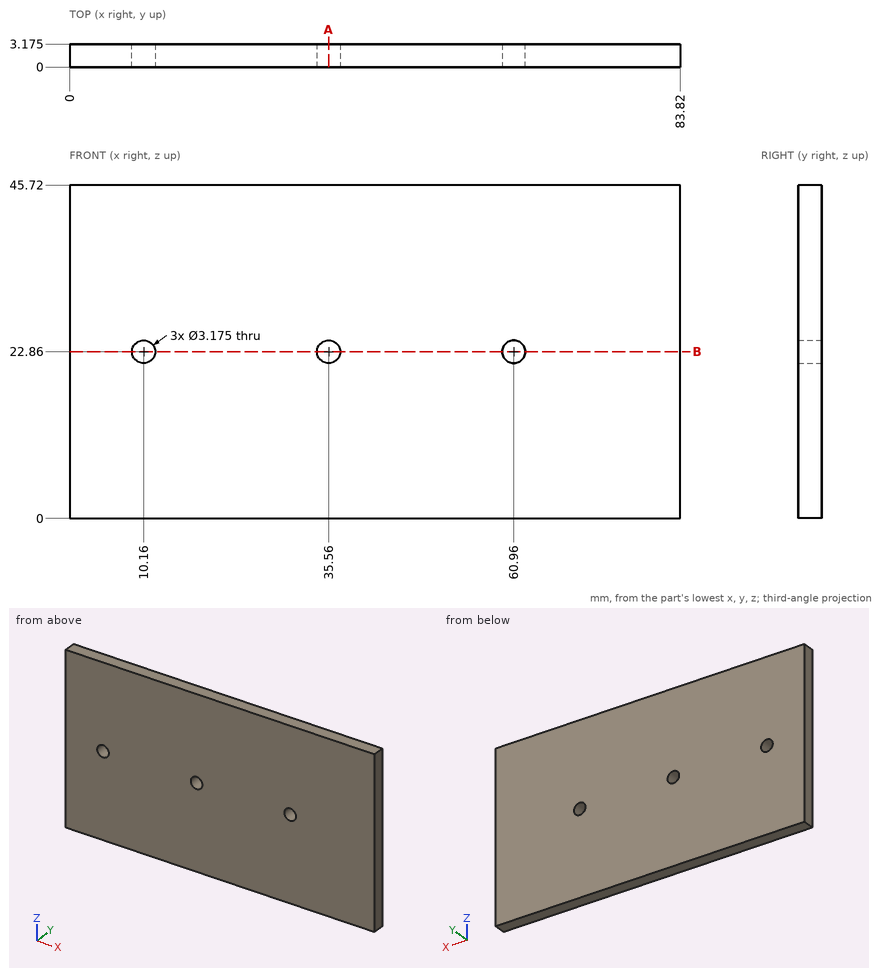
Geometry check sheet. Reference: drawing and pictorial views, mm from the part's lowest x, y, z. Give positions to 0.01 mm unless a question says otherwise; leave off trailing zeros. Write each loop counter-clockwise with the first axis right and the second up, starting at its lowest first coordinate (ties: lowest second). Pieces come first, ordered by that corner, then holes. Notation, with made-up numbers: (18, 42.5) - (28, 42.5) arc R24 ccw to (28, 68.5) - close; hole circle Ø6 at (82.5, 67). An arc over 180 degrees is marked (long way). Use a Markdown table: item, result.
Q1. Section check B-B, the plane z = 22.86. Enter the section's corners in (x, y) (1 decimal), then the cut area to 3 significant figures.
Computed:
| item | result |
|---|---|
| outline | (0, 0) - (8.6, 0) - (8.6, 3.2) - (0, 3.2) - close; (11.7, 0) - (34, 0) - (34, 3.2) - (11.7, 3.2) - close; (37.1, 0) - (59.4, 0) - (59.4, 3.2) - (37.1, 3.2) - close; (62.5, 0) - (83.8, 0) - (83.8, 3.2) - (62.5, 3.2) - close |
| area | 236 mm² |
Q2. Thickness scan on L1, parallel to Z at x = 35.56, y = 1.85. Record the ranges inside material, lowest first. Write a range as [from, to].
Computed:
| item | result |
|---|---|
| L1 | z = [0, 21.27], [24.45, 45.72] |
Q3. Section check A-A, the plane x = 35.56. Enter the section's corners in (y, z) (1 decimal).
Computed:
| item | result |
|---|---|
| outline | (0, 0) - (3.2, 0) - (3.2, 21.3) - (0, 21.3) - close; (0, 24.4) - (3.2, 24.4) - (3.2, 45.7) - (0, 45.7) - close |
Q4. Go/stop test with a flat-tipped pin: P1, Ø3, axis at x = 10.16, z = 22.86, coming from the -Y side. Record where the tip stops, or that it passes through.
Computed:
| item | result |
|---|---|
| P1 | passes through |
